Build history of the part. All positions in model axes, mm. A direction names the side the tool comes from. Give positions to 0.01 mm unless a question says otherwise; leave off trailing zeros. Order: outer loops, then holes, each group sorted by start corner. A loop starts at its lowest first (then second) coordinate and runs counter-clockwise, first axis right, second up. Notation, with made-up numbers: (12, 32.25) - (28, 32.25) arc R10 cw to (28, 38.25) - close; hole circle Ø11 at (30, 3.25). An arc over 180 degrees is marked (long way). One line per item, written item: value.
```python
from build123d import *

# Parameters (mm, degrees)
F1_DEPTH = 17.5
F2_W     = 15
F2_H     = 4
F2_H_2   = 1
F3_DEPTH = 50
F5_DEPTH = 2


with BuildPart() as f1:
    # F0 (on Front) → F1 (new body, symmetric)
    with BuildSketch(Plane.XZ):
        Polygon((-8.5, 0), (0, 0), (8.5, 0), (11.8, 8), (11, 8), (7.75, 2), (0, 2), (-7.75, 2), (-11, 8), (-11.8, 8), align=None)
    extrude(amount=F1_DEPTH, both=True)

    # F2 (on Right) → F3 (cut, symmetric)
    with BuildSketch(Plane.YZ):
        with Locations((0, 4)):
            Rectangle(F2_W, F2_H)
        with Locations((0, 0.5)):
            Rectangle(F2_W, F2_H_2)
    extrude(amount=F3_DEPTH, both=True, mode=Mode.SUBTRACT)

    # F4 (on face) → F5 (join)
    with BuildSketch(Plane(origin=(0, 0, 0), x_dir=(1, 0, 0), z_dir=(0, 0, -1))):
        Polygon((-8.5, 11.780205), (-8.5, 17.5), (-17.5, 22.5), (-17.5, 16.780205), align=None)
        Polygon((-8.5, -11.780205), (-17.5, -16.780205), (-17.5, -22.5), (-8.5, -17.5), align=None)
        Polygon((8.5, -11.780205), (8.5, -17.5), (17.5, -22.5), (17.5, -16.780205), align=None)
        Polygon((17.5, 22.5), (8.5, 17.5), (8.5, 11.780205), (17.5, 16.780205), align=None)
    extrude(amount=-F5_DEPTH)


solid = f1.part
```
(1) Slice it at D-D, the plane y = 18.5. Give the cut face in (x, z), and give its area (3 significant figures).
Completed:
outline: (-17.5, 0) - (-10.3, 0) - (-10.3, 2) - (-17.5, 2) - close; (10.3, 0) - (17.5, 0) - (17.5, 2) - (10.3, 2) - close
area: 28.8 mm²
(2) 3-axis set-ups, long thin cutter, end or side, ignore diameter. For faces 1 (the face through (-13, 20, 1)), 2 (the face through (13.063, 14.315, 0.986)), 3 (the face through (0, 0, 1)), 4 (the face through (0, 17.5, 1)): which of +Z, -Z, +X, -X, +Y, -Y reach the whole face in a straight line?
Completed:
face 1: +Z, -Z, +Y
face 2: -Z, +X
face 3: -Z, +X, -X
face 4: +Z, +Y
(3) Drill centre lines: line 1 (Y direction, x = -10, z = 5.5); line 2 (Z direction, x = 4, y = -13); line 3 (Z direction, x = -8, y = -7). Where is each one in solid material? Low to high.
Completed:
line 1: -17.5 to -7.5, 7.5 to 17.5
line 2: 0 to 2
line 3: 1 to 2
(4) Slice it at B-B, the plane z = 7.25. Give the cut face in (x, y).
Completed:
outline: (-11.49, -17.5) - (-10.59, -17.5) - (-10.59, 17.5) - (-11.49, 17.5) - close; (10.59, -17.5) - (11.49, -17.5) - (11.49, 17.5) - (10.59, 17.5) - close
(5) Slice it at C-C, the plane x = 10.5. Give the cut face in (y, z).
Completed:
outline: (-18.61, 0) - (-12.89, 0) - (-12.89, 2) - (-18.61, 2) - close; (-17.5, 4.85) - (-7.5, 4.85) - (-7.5, 6) - (7.5, 6) - (7.5, 4.85) - (17.5, 4.85) - (17.5, 7.08) - (-17.5, 7.08) - close; (12.89, 0) - (18.61, 0) - (18.61, 2) - (12.89, 2) - close
(6) Pull direction X, two halves, no side cores. Call faces 5 (the face through (10.12, -0.245, 6.375)), 6 (the face through (-12.937, 14.245, 0.986)), 7 (the face through (12.937, -14.245, 0.986)), 8 (the face through (14, -17, 2)): +X half, -X half, draft (parallel to the pull), parting line (faces both ways), or undercut.
Completed:
face 5: undercut
face 6: -X half
face 7: +X half
face 8: draft
(7) Slice it at A-A, the plane y = 2.5. Give the cut face in (x, z) (1 decimal), and give its area (3 significant figures).
Completed:
outline: (-11.8, 8) - (-11, 6) - (-9.9, 6) - (-11, 8) - close; (-9.3, 2) - (-8.9, 1) - (8.9, 1) - (9.3, 2) - close; (9.9, 6) - (11, 6) - (11.8, 8) - (11, 8) - close
area: 22.0 mm²
(8) Pin check, flat tips, straight feed: P1, Ø2, axis at x = -5, z = 1, coming from the +Y side; P2, Ø3, axis at x = 11, y = -4.5, coming from the -Z side; P3, Ø0.8, axis at x = -3.5, z = 0.5, coming from the -Y side. Stop position of each tip, or through.
Completed:
P1: y = 17.5
P2: z = 6
P3: y = -17.5
